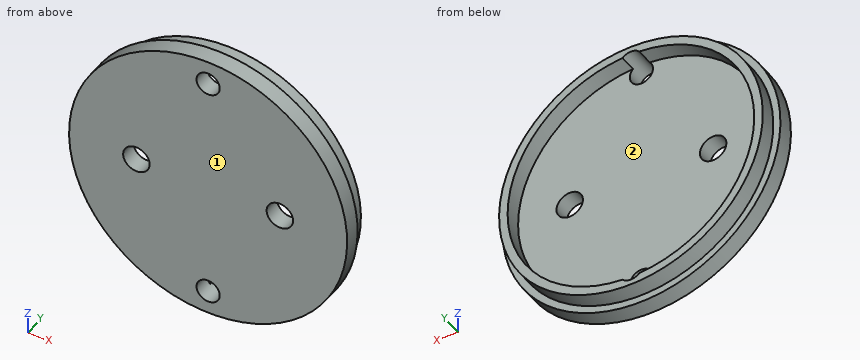
from build123d import *

# Parameters (mm, degrees)
SKETCH1_R               = 38.6
SKETCH1_R_2             = 36.1
BOSS_EXTRUDE1_DEPTH     = 5
SKETCH1_4_R             = 40.7
SKETCH1_4_R_2           = 38.6
SKETCH1_4_R_3           = 36.1
BOSS_EXTRUDE2_DEPTH     = 5
SKETCH4_R               = 3.875
SKETCH4_R_2             = 3.4
CUT_EXTRUDE1_DEPTH      = 59.420715504
CUT_EXTRUDE1_DEPTH_BACK = 59.420715504


with BuildPart() as part:
    # Sketch1 → Boss-Extrude1 (new body)
    with BuildSketch(Plane(origin=(0, 0, 0), x_dir=(1, 0, 0), z_dir=(0, 1, 0))):
        with Locations(Location((0, 0, 0), (0, 0, 270))):
            Circle(SKETCH1_R)
        with Locations(Location((0, 0, 0), (0, 0, 270))):
            Circle(SKETCH1_R_2, mode=Mode.SUBTRACT)
    extrude(amount=BOSS_EXTRUDE1_DEPTH)

    # Sketch1_4 → Boss-Extrude2 (add)
    with BuildSketch(Plane(origin=(0, 0, 0), x_dir=(1, 0, 0), z_dir=(0, 1, 0))):
        with Locations(Location((0, 0, 0), (0, 0, 270))):
            Circle(SKETCH1_4_R)
        with Locations(Location((0, 0, 0), (0, 0, 270))):
            Circle(SKETCH1_4_R_2, mode=Mode.SUBTRACT)
        with Locations(Location((0, 0, 0), (0, 0, 270))):
            Circle(SKETCH1_4_R_2)
        with Locations(Location((0, 0, 0), (0, 0, 270))):
            Circle(SKETCH1_4_R_3, mode=Mode.SUBTRACT)
        with Locations(Location((0, 0, 0), (0, 0, 270))):
            Circle(SKETCH1_4_R_3)
    extrude(amount=-BOSS_EXTRUDE2_DEPTH)

    # Sketch4 → Cut-Extrude1 (cut, two sides)
    with BuildSketch(Plane.XZ.offset(5)) as cut_extrude1_sk:
        with Locations(Location((-21, 0, 0), (0, 0, 90))):
            Circle(SKETCH4_R)
        with Locations(Location((21, 0, 0), (0, 0, 90))):
            Circle(SKETCH4_R)
        with Locations(Location((0, 33.655, 0), (0, 0, 135.994560471))):
            Circle(SKETCH4_R_2)
        with Locations(Location((0, -33.655, 0), (0, 0, 224.005439529))):
            Circle(SKETCH4_R_2)
    extrude(amount=CUT_EXTRUDE1_DEPTH, mode=Mode.SUBTRACT)
    extrude(cut_extrude1_sk.sketch, amount=-CUT_EXTRUDE1_DEPTH_BACK, mode=Mode.SUBTRACT)


solid = part.part
Read the model definition and answer for the solid it produces. Units are mm, in the model's axes. Face numbers are marked on the shaded views. Round coordinates to 2 decimals unless told otherwise and drop trailing zeros. Write each loop counter-clockwise with the first axis right and the second up, starting at its lowest first coordinate (ties: lowest second). Pieces come first, ordered by that corner, then holes. Notation, with made-up numbers: (35.25, -19) - (58.25, -19) arc R33 cw to (58.25, 17) - close; hole circle Ø6 at (33, 58.5). An arc over 180 degrees is marked (long way). One line per question, with ' | ' between items. Start each with the question number.
1. Section C-C (z = -2) is taken. Determine the outline of the cut face in (x, y), and give its area (3 significant figures).
2. Section B-B (y = 3.75) is taken. Determine the outline of the cut face in (x, z) (3 decimals).
3. Section A-A (x = 0) is taken. Determine the outline of the cut face in (y, z) (3 decimals).
4. Each of these flat-tipped pins is pushed along its axis until it touches: pin 1 (6 mm diameter, centred on y = -2, z = 28.5, fed in from -X); pin 2 (8 mm diameter, centred on x = -23, z = -12.5, fed in from +Y); pin 3 (1.5 mm diameter, centred on y = -1, z = 26.5, fed in from -X); pin 4 (7 mm diameter, centred on x = -21, z = 0, fed in from +Y). Where does it stop, or does it pass through?
5. Find the intervals of material crossed by probe 1 along X at (y, z) = (-2.7, 0) (3 decimals); probe 2 along Y at (x, z) = (-13.5, 3); probe 3 along X at (y, z) = (-0.75, 31), in increasing order. Write a range as [from, to].
6. Section D-D (x = -20) is taken. Determine the outline of the cut face in (y, z), and give its area (3 significant figures).
7. For a pull along X with two mould halves and no side action, classify the marked faces 1 and 2 as +X half, -X half, draft (parallel to the pull), parting line (faces both ways), or undercut.
Filled in:
1) outline: (-40.65, -5) - (-24.32, -5) - (-24.32, 0) - (-36.04, 0) - (-36.04, 5) - (-38.55, 5) - (-38.55, 0) - (-40.65, 0) - close; (-17.68, -5) - (17.68, -5) - (17.68, 0) - (-17.68, 0) - close; (24.32, -5) - (40.65, -5) - (40.65, 0) - (38.55, 0) - (38.55, 5) - (36.04, 5) - (36.04, 0) - (24.32, 0) - close | area: 365 mm²
2) outline: circle Ø77.2 at (0, 0); hole (-2.446, -36.017) arc R3.4 ccw to (2.446, -36.017) arc R36.1 ccw to (2.446, 36.017) arc R3.4 ccw to (-2.446, 36.017) arc R36.1 ccw to start
3) outline: (-5, -40.7) - (0, -40.7) - (0, -38.6) - (5, -38.6) - (5, -37.055) - (-5, -37.055) - close; (-5, -30.255) - (0, -30.255) - (0, 30.255) - (-5, 30.255) - close; (-5, 37.055) - (5, 37.055) - (5, 38.6) - (0, 38.6) - (0, 40.7) - (-5, 40.7) - close
4) pin 1: x = -31.72 | pin 2: y = 0 | pin 3: x = -31.52 | pin 4: through
5) probe 1: [-40.7, -24.875], [-17.125, 17.125], [24.875, 40.7] | probe 2: [-5, 0] | probe 3: [-26.37, -2.12], [2.12, 26.37]
6) outline: (-5, -35.45) - (0, -35.45) - (0, -33.01) - (5, -33.01) - (5, -30.05) - (0, -30.05) - (0, -3.74) - (-5, -3.74) - close; (-5, 3.74) - (0, 3.74) - (0, 30.05) - (5, 30.05) - (5, 33.01) - (0, 33.01) - (0, 35.45) - (-5, 35.45) - close | area: 347 mm²
7) face 1: draft | face 2: undercut
